Source: CAD feature listing. Evaluate the final solid. Frame: model axes, mm. A direction names the side the tool comes from. Give positions to 0.01 mm unless a question says otherwise; leave off trailing zeros. Order: outer loops, then holes, each group sorted by start corner. A loop starts at its lowest first (then second) coordinate and runs counter-clockwise, first axis right, second up. Notation, with made-up numbers: M 64,75 L 99,75 A13 cw 99,100 Z; hole C -36.75,40 d11. An arc over 180 degrees is marked long. Answer as a JSON object with one key per item and string values. Group by question number.
1. Pin query (flat end, axial travel): P1, Ø21.5, axis at x = 38.5, y = -15.5, coming from the +Z side; P2, Ø5, axis at x = 35, z = 13, coming from the -Y side. Return the tip coordinate at first contact, or that it passes through.
2. Section query B-B (x = 7). Output: boundary loops of the cut face in (y, z), plus the area to 3 significant figures.
3. Material intervals for L1, parallel to Z at x = 10, y = -9; L2, parallel to Y at x = 26, z = 19.5, sorted ascending. Write a range as [from, to].
4. Set-up query: faces 1 (the flat face through (14, 0, 13)), 2 (the flat face through (20, -17, 0.254)). Return all of +Z, -Z, +X, -X, +Y, -Y with unobstructed straight access to the full face (end or side cutting, diameter ignored); none if empty.
5. Section query A-A (y = -25.5). Output: boundary loops of the cut face in (x, z), plus the area to 3 significant figures.
from build123d import *

# Parameters (mm, degrees)
F1_DEPTH = 0.254
F3_DEPTH = 0.254
F5_DEPTH = 0.254


with BuildPart() as f1:
    # F0 (on Front) → F1 (new body)
    with BuildSketch(Plane.XZ):
        Polygon((0, 44.969123), (0, 0), (52.707318, 0), align=None)
    extrude(amount=F1_DEPTH)

    # F2 (on Right) → F3 (join)
    with BuildSketch(Plane.YZ):
        Polygon((-44.229742, 0), (0, 0), (0, 44.73836), align=None)
    extrude(amount=F3_DEPTH)

    # F4 (on Top) → F5 (join)
    with BuildSketch(Plane.XY):
        Polygon((0, 0), (0, -43.801095), (52.415315, 0), align=None)
    extrude(amount=F5_DEPTH)


solid = f1.part
Answer sheet:
{
 "1": {"P1": "z = 0.25", "P2": "y = -0.25"},
 "2": {"outline": "M -37.95,0 L 0,0 L 0,39 L -0.25,39 L -0.25,0.25 L -37.95,0.25 Z", "area": "19.5 mm^2"},
 "3": {"L1": "[0, 0.25]", "L2": "[-0.25, 0]"},
 "4": {"face 1": "+Z, -Z, +X, -X, +Y", "face 2": "+Z, +X, -Y"},
 "5": {"outline": "M 0,0 L 21.9,0 L 21.9,0.25 L 0.25,0.25 L 0.25,18.95 L 0,18.95 Z", "area": "10.3 mm^2"}
}
